from build123d import *

# Parameters (mm, degrees)
SKETCH_1_R          = 16.5
EXTRUDE_1_DEPTH     = 2.5
SKETCH_2_R          = 33.5
EXTRUDE_2_DEPTH     = 32
SKETCH_3_R          = 11
EXTRUDE_3_DEPTH     = 10
SKETCH_4_R          = 1.5
CUT_EXTRUDE_1_DEPTH = 5
SKETCH_5_R          = 1.5
CUT_EXTRUDE_2_DEPTH = 5


with BuildPart() as part:
    # 草图1 → 凸台-拉伸1 (new body)
    with BuildSketch(Plane.XY):
        Circle(SKETCH_1_R)
    extrude(amount=EXTRUDE_1_DEPTH)

    # 草图2 → 凸台-拉伸2 (add)
    with BuildSketch(Plane.XY.offset(2.5)):
        Circle(SKETCH_2_R)
    extrude(amount=EXTRUDE_2_DEPTH)

    # 草图3 → 凸台-拉伸3 (add)
    with BuildSketch(Plane.XY.offset(34.5)):
        Circle(SKETCH_3_R)
    extrude(amount=EXTRUDE_3_DEPTH)

    # 草图4 → 切除-拉伸1 (cut)
    with BuildSketch(Plane.XY.offset(44.5)):
        with Locations((7.577722283, 4.375)):
            Circle(SKETCH_4_R)
        with Locations((-7.577722283, 4.375)):
            Circle(SKETCH_4_R)
        with Locations((0, -8.75)):
            Circle(SKETCH_4_R)
    extrude(amount=-CUT_EXTRUDE_1_DEPTH, mode=Mode.SUBTRACT)

    # 草图5 → 切除-拉伸2 (cut)
    with BuildSketch(Plane(origin=(0, 0, 0), x_dir=(-1, 0, 0), z_dir=(0, 0, -1))):
        with Locations((0, -14)):
            Circle(SKETCH_5_R)
        with Locations((-12.124355653, 7)):
            Circle(SKETCH_5_R)
        with Locations((12.124355653, 7)):
            Circle(SKETCH_5_R)
    extrude(amount=-CUT_EXTRUDE_2_DEPTH, mode=Mode.SUBTRACT)


solid = part.part
Could you check a few things on this model? Use its own coordinates, in mm. A direction names the side the tool comes from. Coordinates: 2 decimals unless noted, no trailing zeros. Write each loop counter-clockwise with the first axis right and the second up, starting at its lowest first coordinate (ties: lowest second). Pieces come first, ordered by that corner, then holes. Notation, with made-up numbers: (51.5, 53) - (77.5, 53) arc R8 cw to (77.5, 68) - close; hole circle Ø7 at (79, 46). An arc over 180 degrees is marked (long way). Put each result on its own line as item: value. Start each with the question number.
Q1. Please list where these lines run through material, in increasing order: L1, parallel to Y at x = 0, z = 40.7; L2, parallel to Z at x = -13, y = 12.5; L3, parallel to X at y = -8.5, z = 40.5.
Q2. Which directions (+Z, -Z, +X, -X, +Y, -Y) give clear straight access to the entire face, cutting with the end or side of a thin tool? Please do faces 1 (the cylindrical face through (-6.192, 3.8, 42.035)), 2 (the flat face through (0, 0, 0)), 3 (the flat face through (-15.4, -7, 2.5)).
Q3. I'm going to push flat-ended pins straight in: P1, Ø2.5, axis at x = -12.12, y = 7, coming from the -Z side; P2, Ø10, axis at x = 3.5, y = 15.5, coming from the +Z side; P3, Ø0.9, axis at x = -7.5, y = 4.5, coming from the +Z side; P4, Ø1, axis at x = -6, z = 27, coming from the -Y side. Where does each tip first touch, or does it pass through?
Q4. I want a section at B-B on y = 0. Write out the boundary of the cut face in (x, z), plus the area to 3 significant figures.
Q5. I want a section at A-A on x = 0. Write out the boundary of the cut face in (y, z).
Q6. Thinking about a two-plate mould opening in Y: for faces 4 (the cylindrical face through (11.43, 5.67, 2.46)), 5 (the flat face through (-8, 8, 34.5)), 6 (the cylindrical face through (-2.38, -10.74, 39.43)), which applies, pulls with the +Y half, pulls with the -Y half, needs draft (parallel to the pull), parting line crosses it, or undercut?
Q7. I want a section at C-C on z = 38. Write out the boundary of the cut face in (x, y), plus the area to 3 significant figures.
Q8. I want a section at D-D on y = 7. Write out the boundary of the cut face in (x, z), plus the area to 3 significant figures.
Checks:
1. L1: -11 to -10.25, -7.25 to 11
1. L2: 2.5 to 34.5
1. L3: -6.98 to -1.48, 1.48 to 6.98
2. face 1: +Z
2. face 2: -Z, +X, -X, +Y, -Y
2. face 3: -Z
3. P1: z = 5
3. P2: z = 44.5
3. P3: z = 39.5
3. P4: y = -33.05
4. outline: (-33.5, 2.5) - (-16.5, 2.5) - (-16.5, 0) - (16.5, 0) - (16.5, 2.5) - (33.5, 2.5) - (33.5, 34.5) - (11, 34.5) - (11, 44.5) - (-11, 44.5) - (-11, 34.5) - (-33.5, 34.5) - close
4. area: 2,450 mm²
5. outline: (-33.5, 2.5) - (-16.5, 2.5) - (-16.5, 0) - (-15.5, 0) - (-15.5, 5) - (-12.5, 5) - (-12.5, 0) - (16.5, 0) - (16.5, 2.5) - (33.5, 2.5) - (33.5, 34.5) - (11, 34.5) - (11, 44.5) - (-7.25, 44.5) - (-7.25, 39.5) - (-10.25, 39.5) - (-10.25, 44.5) - (-11, 44.5) - (-11, 34.5) - (-33.5, 34.5) - close
6. face 4: undercut
6. face 5: needs draft
6. face 6: parting line crosses it
7. outline: circle Ø22 at (0, 0)
7. area: 380 mm²
8. outline: (-32.76, 2.5) - (-14.94, 2.5) - (-14.94, 0) - (-13.62, 0) - (-13.62, 5) - (-10.62, 5) - (-10.62, 0) - (10.62, 0) - (10.62, 5) - (13.62, 5) - (13.62, 0) - (14.94, 0) - (14.94, 2.5) - (32.76, 2.5) - (32.76, 34.5) - (8.49, 34.5) - (8.49, 44.5) - (-8.49, 44.5) - (-8.49, 34.5) - (-32.76, 34.5) - close
8. area: 2,310 mm²
